```python
from build123d import *

# Parameters (mm, degrees)
F0_R          = 5.373622476
F1_DEPTH      = 215.88753
F3_DEPTH      = 2.54
F3_DEPTH_BACK = 2.54
F4_T2_ANGLE   = 126.5345537541
F4_T4_ANGLE   = 126.5345537541


# Not quite as in the source:
# - a fillet or chamfer that OpenCascade refuses, or shapes differently, is made with other operations: its cross-section is extruded or revolved along the edge and cut away or added


with BuildPart() as f1:
    # F0 (on Front) → F1 (new body)
    with BuildSketch(Plane.XZ):
        Circle(F0_R)
    extrude(amount=F1_DEPTH)

    # F2 (on Top) → F3 (join, two sides)
    with BuildSketch(Plane.XY) as f3_sk:
        Polygon((-8.9527533501, 1.9022722074), (-4.8790749139, 1.0367010286), (-6.158160232, 3.4090294491), align=None)
        Polygon((-13.7193289536, 2.9150694934), (-8.9527533501, 1.9022722074), (-10.4493999233, 4.6781129985), align=None)
        Polygon((-18.2748671635, 3.8830257621), (-13.7193289536, 2.9150694934), (-15.1497123605, 5.5680115299), align=None)
        Polygon((-22.0207331241, 4.6789436692), (-18.2748671635, 3.8830257621), (-19.4510233645, 6.0644508345), align=None)
        Polygon((-25.0378297706, 5.3200133908), (-22.0207331241, 4.6789436692), (-22.9680646536, 6.4359660347), align=None)
        Polygon((-27.890320124, 5.9261077295), (-25.0378297706, 5.3200133908), (-25.9334769328, 6.9811764013), align=None)
        Polygon((-28.7897214748, 7.5942336596), (-30.7547669567, 6.5347425691), (-27.890320124, 5.9261077295), align=None)
        Polygon((-32.1493126453, 9.1212161407), (-35.1961678702, 7.4784470575), (-30.7547669567, 6.5347425691), align=None)
        Polygon((-35.1961678702, 9.5456602661), (-37.6418792182, 7.9981093941), (-35.1961678702, 7.4784470575), align=None)
        Polygon((-38.8515780683, 9.9098877134), (-40.8092972733, 8.6711192604), (-37.6418792182, 7.9981093941), align=None)
        Polygon((-42.7175686579, 11.6869044373), (-45.8058244977, 9.7327764402), (-40.8092972733, 8.6711192604), align=None)
        Polygon((-47.1321087681, 11.8288034913), (-49.2785042842, 10.4706480183), (-45.8058244977, 9.7327764402), align=None)
        Polygon((-50.8480016213, 12.9510430201), (-53.3880016213, 11.343829962), (-49.2785042842, 10.4706480183), align=None)
        Polygon((-2.9497377109, 0), (0, 0), (-2.9497377109, 0.6267573614), align=None)
        Polygon((1.198072837, 19.0015498009), (3.3619815949, 13.447928708), (3.3619815949, 25.0585451722), align=None)
        Polygon((3.0523012392, 22.8999685496), (3.0523012392, 15.3504825952), (1.7903243424, 18.9260840416), align=None, mode=Mode.SUBTRACT)
        Polygon((-4.2252911557, 24.8437412083), (-4.2252911557, 13.2858192763), (-1.4181542095, 19.1259601465), align=None)
        Polygon((-3.7408936769, 22.9805186391), (-2.2895061411, 19.10783723), (-3.7408936769, 15.6503133476), align=None, mode=Mode.SUBTRACT)
        Polygon((-2.9497377109, 0.6267573614), (0, 0), (2.1719516162, 0), (2.1719516162, 7.62), (5.6152132711, 7.6650624399), (3.3619815949, 13.447928708), (1.198072837, 19.0015498009), (0, 22.0763756473), (-1.4181542095, 19.1259601465), (-4.2252911557, 13.2858192763), (-6.9486382417, 7.62), (-2.9497377109, 7.62), align=None)
        Polygon((-2.9854448512, 13.0213079974), (-2.9854448512, 8.1413947046), (-5.9038246982, 8.1413947046), (-2.9854448512, 14.2129721679), align=None, mode=Mode.SUBTRACT)
        Polygon((2.1099960018, 14.3143812405), (4.47795121, 8.2370797172), (2.1719516162, 8.2069007827), (2.1089701391, 13.0193722181), align=None, mode=Mode.SUBTRACT)
        Polygon((-2.2104110103, 15.9188192338), (0, 20.6176694483), (1.7634738469, 15.9993711859), (0, 11.8375318125), align=None, mode=Mode.SUBTRACT)
        with BuildLine():
            Line((-34.7528146772, -32.0806060351), (-34.7528146772, -20.9908965406))
            Line((-34.7528146772, -20.9908965406), (0, -14.0988837661))
            Line((0, -14.0988837661), (0, 0))
            Line((0, 0), (-2.9497377109, 0))
            Line((-2.9497377109, 0), (-2.9497377109, 0.6267573614))
            Line((-2.9497377109, 0.6267573614), (-4.8790749139, 1.0367010286))
            Line((-4.8790749139, 1.0367010286), (-8.9527533501, 1.9022722074))
            Line((-8.9527533501, 1.9022722074), (-13.7193289536, 2.9150694934))
            Line((-13.7193289536, 2.9150694934), (-18.2748671635, 3.8830257621))
            Line((-18.2748671635, 3.8830257621), (-22.0207331241, 4.6789436692))
            Line((-22.0207331241, 4.6789436692), (-25.0378297706, 5.3200133908))
            Line((-25.0378297706, 5.3200133908), (-27.890320124, 5.9261077295))
            Line((-27.890320124, 5.9261077295), (-30.7547669567, 6.5347425691))
            Line((-30.7547669567, 6.5347425691), (-35.1961678702, 7.4784470575))
            Line((-35.1961678702, 7.4784470575), (-37.6418792182, 7.9981093941))
            Line((-37.6418792182, 7.9981093941), (-40.8092972733, 8.6711192604))
            Line((-40.8092972733, 8.6711192604), (-45.8058244977, 9.7327764402))
            Line((-45.8058244977, 9.7327764402), (-49.2785042842, 10.4706480183))
            Line((-49.2785042842, 10.4706480183), (-53.3880016213, 11.343829962))
            Line((-53.3880016213, 11.343829962), (-54.9966600991, 11.6856361297))
            ThreePointArc((-54.9966600991, 11.6856361297), (-66.0747003656, -11.2262862037), (-55.3715413676, -34.3157112426))
            Line((-55.3715413676, -34.3157112426), (-34.7528146772, -32.0806060351))
        make_face()
        with BuildLine():
            ThreePointArc((-51.421571523, -31.2265530229), (-63.6234506771, -11.4887260787), (-53.1807132065, 9.2336507514))
            Line((-53.1807132065, 9.2336507514), (-51.5400195681, 7.2946498786))
            ThreePointArc((-51.5400195681, 7.2946498786), (-61.3618234836, -11.493283063), (-50.339024514, -29.6027325094))
            Line((-50.339024514, -29.6027325094), (-51.421571523, -31.2265530229))
        make_face(mode=Mode.SUBTRACT)
        Polygon((-49.3917986751, -26.8963649869), (-49.256477505, 5.174099002), (-46.8207485974, 5.174099002), (-46.8207485974, -26.8963649869), align=None, mode=Mode.SUBTRACT)
        Polygon((-42.3252023757, 3.8717763964), (-8.7594440334, -1.5370512847), (-8.7594440334, -13.9601901174), (-42.3252023757, -13.9601901174), (-42.3252023757, -1.5370512847), align=None, mode=Mode.SUBTRACT)
    extrude(amount=F3_DEPTH)
    extrude(f3_sk.sketch, amount=-F3_DEPTH_BACK)

    # F4: chamfer of 2.54 on 2 edges, made by hand

    # F4_s1 → F4_t2 (revolve, cut)
    with BuildSketch(Plane(origin=(-33.7752745406, -16.6677099753, 0), x_dir=(0, 0, 1), z_dir=(0.8967506648, 0.4425361512, 0))):
        Polygon((0, -35.5324348562), (2.54, -32.9924348562), (2.54, -35.5324348562), align=None)
    revolve(axis=Axis((-36.340977144, -11.4685968428, 2.54), (0, 0, 1)), revolution_arc=F4_T2_ANGLE, mode=Mode.SUBTRACT)

    # F4_s3 → F4_t4 (revolve, cut)
    with BuildSketch(Plane(origin=(-33.7752745406, -16.6677099753, 0), x_dir=(0, 0, 1), z_dir=(0.8967506648, 0.4425361512, 0))):
        Polygon((-2.54, -32.9924348562), (0, -35.5324348562), (-2.54, -35.5324348562), align=None)
    revolve(axis=Axis((-36.340977144, -11.4685968428, -2.54), (0, 0, 1)), revolution_arc=F4_T4_ANGLE, mode=Mode.SUBTRACT)


solid = f1.part
```
Check sheet for the modelled part. Datum: model origin and axes. Units: mm. A direction names the side the tool comes from. Coordinates: 2 decimals unless noted, no trailing zeros. Write each loop counter-clockwise with the first axis right and the second up, starting at its lowest first coordinate (ties: lowest second). Pieces come first, ordered by that corner, then holes. Notation, with made-up numbers: M 29,33.25 L 46,33.25 A21 ccw 46,45.25 Z; hole C -29,33.5 d7. An arc over 180 degrees is marked long. Write item = value, one per line. Start each with the question number.
1. Go/stop test with flat-tipped pins: pin 1 (4 mm diameter, centred on y = 10.5, z = -0.5, fed in from -X); pin 2 (5.5 mm diameter, centred on y = 19.5, z = 1, fed in from -X); pin 3 (6 mm diameter, centred on y = -61.5, z = -3, fed in from -X). Record where each tip stops, or that it passes through.
2. Sectioned sample at A-A (y = -196). Record the cut outline in (x, z), then the cut area to 3 significant figures.
3. Thickness scan on probe 1 along Y at (x, z) = (-57.5, 1.25); probe 2 along X at (y, z) = (-192, 0.25); probe 3 along Y at (x, z) = (-57, -2.25). Record the ranges inside material, lowest first.
4. Mould release check, pull along Y, two halves, no side actions. Record for faces 4 (the flat face through (-19.954, -18.056, 0.036)), 5 (the cylindrical face through (-61.37, -11.18, 0.04)), 6 (the flat face through (-5.57, 10.49, 0.04)): pulls with the +Y half, pulls with the -Y half, needs draft (parallel to the pull), parting line crosses it, or undercut.
5. Tool access check on faces 1 (the flat face through (-2.95, 4, 0)), 2 (the flat face through (-45.207, -33.214, 0.036)), 3 (the flat face through (3.362, 19, 0)). Record the directions out of +Z, -Z, +X, -X, +Y, -Y that give a thin tool (end or side, any length) a straight path to the whole face; none if there is none.
The answers:
q1.pin_1 = -58.32
q1.pin_2 = -4.23
q1.pin_3 = -5.37
q2.outline = C 0,0 d10.75
q2.area = 90.7 mm²
q3.probe_1 = -30.54 to -26.4, -23.12 to 1.53, 5.49 to 7.6
q3.probe_2 = -5.37 to 5.37
q3.probe_3 = -29.6 to -26.94, -23.81 to 2.22, 6.02 to 6.66
q4.face_4 = pulls with the -Y half
q4.face_5 = undercut
q4.face_6 = pulls with the +Y half
q5.face_1 = +Z, -Z
q5.face_2 = +Z, -Z, -Y
q5.face_3 = +Z, -Z, +X, +Y
